For this review, use the dimensioned drawing (mm, ordinates from the lowest corner) and the shaded views. Round coordinates to 2 decimals unless told otherwise and drop trailing zeros. Loops run counter-clockwise (first coordinate to the right, second up) from the corner with the lowest first, then second, coordinate; pieces in that order, holes last.
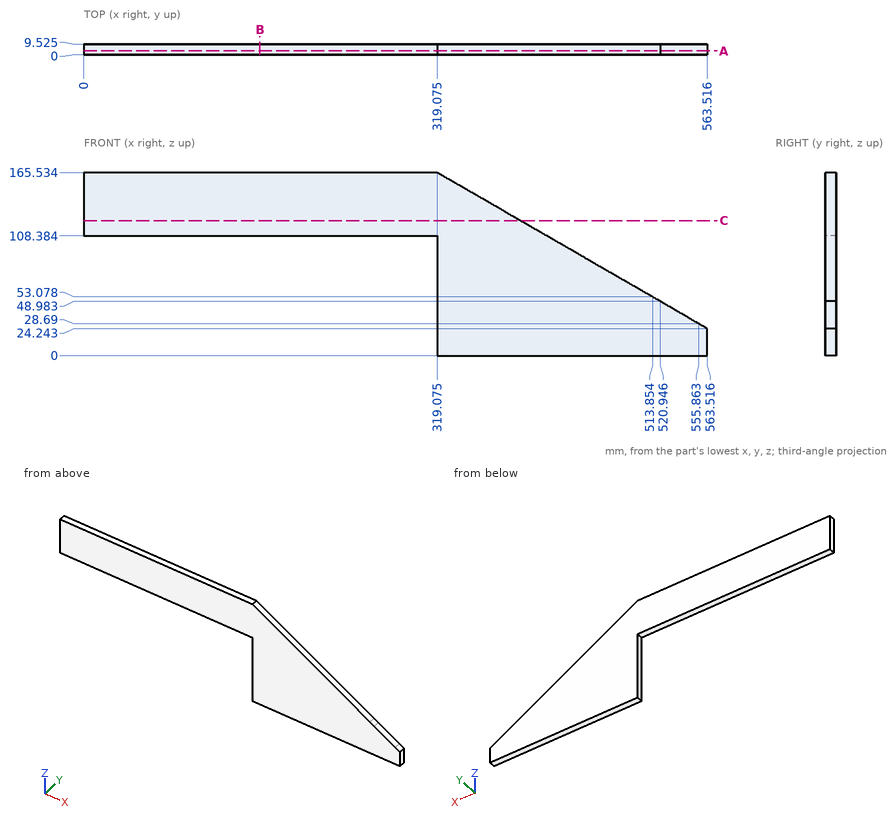
(1) Add section A-A (y = 3.25). Give the boundary of the cut face in (x, z) (1 decimal), plus the area to 3 significant figures.
(2) For L1, parallel to Z at x = 170, y = 8.75; L2, parallel to X at y = 8.25, z = 7 (1 decimal); L3, parallel to X at y = 4.75, z = 65 (1 decimal), list the stretches that pass through material, from the lowest coordinate up.
(3) Insertion check: pin 1 Ø2 at (y, z) = (8, 92) entering from +X; pin 2 Ø1 at (y, z) = (3, 31) entering from +X; pin 3 Ø3 at (x, y) = (141, 5) entering from -Z. Each pin has a flat end and moves straight along its axis. Give the tip position at first contact, or say it passes through.
(4) Add section B-B (x = 159). Give the boundary of the cut face in (y, z) (1 decimal).
(5) Add section C-C (z = 122). Give the boundary of the cut face in (x, y) (1 decimal), plus the area to 3 significant figures.
Outcome:
1. outline: (0, 108.4) - (319.1, 108.4) - (319.1, 0) - (563.5, 0) - (563.5, 24.2) - (520.9, 49) - (319.1, 165.5) - (0, 165.5) - close
1. area: 41,400 mm2
2. L1: z = 108.38 to 165.53
2. L2: x = 319.1 to 563.5
2. L3: x = 319.1 to 493.2
3. pin 1: stops at x = 448.17
3. pin 2: stops at x = 552.75
3. pin 3: stops at z = 108.38
4. outline: (0, 108.4) - (9.5, 108.4) - (9.5, 165.5) - (0, 165.5) - close
5. outline: (0, 0) - (394.5, 0) - (394.5, 9.5) - (0, 9.5) - close
5. area: 3,760 mm2
